```python
from build123d import *

# Parameters (mm, degrees)
SKETCH1_R           = 32.5
SKETCH1_R_2         = 1.0625
BOSS_EXTRUDE1_DEPTH = 4.5
SCALE1_SCALE        = 25.4


with BuildPart() as part:
    # Sketch1 → Boss-Extrude1 (new body)
    with BuildSketch(Plane.XY):
        Circle(SKETCH1_R)
        with Locations((0, 30.375)):
            Circle(SKETCH1_R_2, mode=Mode.SUBTRACT)
        with Locations((4.751696876, 30.001033346)):
            Circle(SKETCH1_R_2, mode=Mode.SUBTRACT)
        with Locations((9.386391204, 28.888341682)):
            Circle(SKETCH1_R_2, mode=Mode.SUBTRACT)
        with Locations((13.78996143, 27.064323172)):
            Circle(SKETCH1_R_2, mode=Mode.SUBTRACT)
        with Locations((17.853977038, 24.573891204)):
            Circle(SKETCH1_R_2, mode=Mode.SUBTRACT)
        with Locations((21.478368479, 21.478368479)):
            Circle(SKETCH1_R_2, mode=Mode.SUBTRACT)
        with Locations((24.573891204, 17.853977038)):
            Circle(SKETCH1_R_2, mode=Mode.SUBTRACT)
        with Locations((27.064323172, 13.78996143)):
            Circle(SKETCH1_R_2, mode=Mode.SUBTRACT)
        with Locations((28.888341682, 9.386391204)):
            Circle(SKETCH1_R_2, mode=Mode.SUBTRACT)
        with Locations((30.001033346, 4.751696876)):
            Circle(SKETCH1_R_2, mode=Mode.SUBTRACT)
        with Locations((30.375, 0)):
            Circle(SKETCH1_R_2, mode=Mode.SUBTRACT)
        with Locations((30.001033346, -4.751696876)):
            Circle(SKETCH1_R_2, mode=Mode.SUBTRACT)
        with Locations((28.888341682, -9.386391204)):
            Circle(SKETCH1_R_2, mode=Mode.SUBTRACT)
        with Locations((27.064323172, -13.78996143)):
            Circle(SKETCH1_R_2, mode=Mode.SUBTRACT)
        with Locations((24.573891204, -17.853977038)):
            Circle(SKETCH1_R_2, mode=Mode.SUBTRACT)
        with Locations((21.478368479, -21.478368479)):
            Circle(SKETCH1_R_2, mode=Mode.SUBTRACT)
        with Locations((17.853977038, -24.573891204)):
            Circle(SKETCH1_R_2, mode=Mode.SUBTRACT)
        with Locations((13.78996143, -27.064323172)):
            Circle(SKETCH1_R_2, mode=Mode.SUBTRACT)
        with Locations((9.386391204, -28.888341682)):
            Circle(SKETCH1_R_2, mode=Mode.SUBTRACT)
        with Locations((4.751696876, -30.001033346)):
            Circle(SKETCH1_R_2, mode=Mode.SUBTRACT)
        with Locations((0, -30.375)):
            Circle(SKETCH1_R_2, mode=Mode.SUBTRACT)
        with Locations((-4.751696876, -30.001033346)):
            Circle(SKETCH1_R_2, mode=Mode.SUBTRACT)
        with Locations((-9.386391204, -28.888341682)):
            Circle(SKETCH1_R_2, mode=Mode.SUBTRACT)
        with Locations((-13.78996143, -27.064323172)):
            Circle(SKETCH1_R_2, mode=Mode.SUBTRACT)
        with Locations((-17.853977038, -24.573891204)):
            Circle(SKETCH1_R_2, mode=Mode.SUBTRACT)
        with Locations((-21.478368479, -21.478368479)):
            Circle(SKETCH1_R_2, mode=Mode.SUBTRACT)
        with Locations((-24.573891204, -17.853977038)):
            Circle(SKETCH1_R_2, mode=Mode.SUBTRACT)
        with Locations((-27.064323172, -13.78996143)):
            Circle(SKETCH1_R_2, mode=Mode.SUBTRACT)
        with Locations((-28.888341682, -9.386391204)):
            Circle(SKETCH1_R_2, mode=Mode.SUBTRACT)
        with Locations((-30.001033346, -4.751696876)):
            Circle(SKETCH1_R_2, mode=Mode.SUBTRACT)
        with Locations((-30.375, 0)):
            Circle(SKETCH1_R_2, mode=Mode.SUBTRACT)
        with Locations((-30.001033346, 4.751696876)):
            Circle(SKETCH1_R_2, mode=Mode.SUBTRACT)
        with Locations((-28.888341682, 9.386391204)):
            Circle(SKETCH1_R_2, mode=Mode.SUBTRACT)
        with Locations((-27.064323172, 13.78996143)):
            Circle(SKETCH1_R_2, mode=Mode.SUBTRACT)
        with Locations((-24.573891204, 17.853977038)):
            Circle(SKETCH1_R_2, mode=Mode.SUBTRACT)
        with Locations((-21.478368479, 21.478368479)):
            Circle(SKETCH1_R_2, mode=Mode.SUBTRACT)
        with Locations((-17.853977038, 24.573891204)):
            Circle(SKETCH1_R_2, mode=Mode.SUBTRACT)
        with Locations((-13.78996143, 27.064323172)):
            Circle(SKETCH1_R_2, mode=Mode.SUBTRACT)
        with Locations((-9.386391204, 28.888341682)):
            Circle(SKETCH1_R_2, mode=Mode.SUBTRACT)
        with Locations((-4.751696876, 30.001033346)):
            Circle(SKETCH1_R_2, mode=Mode.SUBTRACT)
    extrude(amount=BOSS_EXTRUDE1_DEPTH)


with BuildPart() as part_1:
    # Scale1: scaled about (0, 0, 2.25)
    add(part.part.scale(SCALE1_SCALE).moved(Location((0, 0, -54.9))))


solid = part_1.part
```
Can you work these out from the model? Positions are in its coordinate system, mm. Coordinates: 2 decimals unless noted, no trailing zeros. Loops run counter-clockwise (first coordinate to the right, second up) from the corner with the lowest first, then second, coordinate; pieces in that order, holes last. Notation, with made-up numbers: (11.25, -16) -> (32.25, -16) arc R11 ccw to (32.25, -11) -> close; hole circle Ø9 at (9.5, 34). An arc over 180 degrees is marked (long way). Put each result on its own line as item: value. Start each with the question number.
Q1. I'm going to push flat-ended pins straight in: P1, Ø1.5, axis at y = 69, z = 24.5, coming from the -X side; P2, Ø1, axis at x = -244, z = -18, coming from the -Y side; P3, Ø8, axis at y = 421, z = 39.5, coming from the +X side. Where does each tip first touch, or does it pass through?
Q2. If I drill on line 1 (Y direction, x = 0, z = 23); line 2 (Y direction, x = 96, z = -5); line 3 (X direction, y = 437.5, z = -12.5), over which ranges is the centre line in solid material (lowest first)? Write a range as [from, to].
Q3. I want a section at C-C (z = 3). Count the separate pieces of the cut face and the enclosed holes in it, plus the area to 3 significant figures.
Q4. I want a section at A-A (y = 0). Write out the boundary of the cut face in (x, z), plus the area to 3 significant figures.
Q5. Thinking about a two-plate mould opening in X: for faces 1 (the face through (-244.3, -760.1, 1.4)), 2 (the face through (-12, 12, 59.4)), which applies, pulls with the +X half, pulls with the -X half, needs draft (parallel to the pull), parting line crosses it, or undercut?
Taken from the geometry:
1. P1: stops at x = -822.67
1. P2: stops at y = -788.77
1. P3: stops at x = 712.43
2. line 1: y = [-825.5, -798.51], [-744.54, 744.54], [798.51, 825.5]
2. line 2: y = [-819.9, -772.92], [-751.14, 751.14], [772.92, 819.9]
2. line 3: x = [-700.03, -645.92], [-602.44, 602.44], [645.92, 700.03]
3. separate pieces: 1
3. enclosed holes: 40
3. area: 2,050,000 mm2
4. outline: (-825.5, -54.9) -> (-798.51, -54.9) -> (-798.51, 59.4) -> (-825.5, 59.4) -> close; (-744.54, -54.9) -> (744.54, -54.9) -> (744.54, 59.4) -> (-744.54, 59.4) -> close; (798.51, -54.9) -> (825.5, -54.9) -> (825.5, 59.4) -> (798.51, 59.4) -> close
4. area: 176,000 mm2
5. face 1: undercut
5. face 2: needs draft
